```python
from build123d import *

# Parameters (mm, degrees)
SKETCH1_W           = 50
SKETCH1_H           = 9
SKETCH1_W_2         = 9
SKETCH1_H_2         = 68
BOSS_EXTRUDE1_DEPTH = 28
SKETCH2_R           = 2.5
CUT_EXTRUDE2_DEPTH  = 100
SKETCH4_R           = 4.5
CUT_EXTRUDE3_DEPTH  = 10
SKETCH5_R           = 10
CUT_EXTRUDE4_DEPTH  = 6
SKETCH7_R           = 1.5
CUT_EXTRUDE5_DEPTH  = 10
CUT_EXTRUDE6_DEPTH  = 10


with BuildPart() as part:
    # Sketch1 → Boss-Extrude1 (new body)
    with BuildSketch(Plane.XY):
        with Locations((-32.879310345, 31.301724138)):
            Rectangle(SKETCH1_W, SKETCH1_H)
        with Locations((-3.379310345, 1.801724138)):
            Rectangle(SKETCH1_W_2, SKETCH1_H_2)
        with Locations((-32.879310345, -27.698275862)):
            Rectangle(SKETCH1_W, SKETCH1_H)
    extrude(amount=BOSS_EXTRUDE1_DEPTH)

    # Sketch2 → Cut-Extrude2 (cut)
    with BuildSketch(Plane(origin=(0, 35.801724138, 0), x_dir=(1, 0, 0), z_dir=(0, 1, 0))):
        with Locations(Location((-43.879310345, -14, 0), (0, 0, 180))):
            Circle(SKETCH2_R)
        with BuildLine():
            ThreePointArc((-43.879310345, -28), (-53.778805281, -23.899494937), (-57.879310345, -14))
            Line((-57.879310345, -14), (-57.879310345, -28))
            Line((-57.879310345, -28), (-43.879310345, -28))
        make_face()
        with BuildLine():
            Line((-57.879310345, 0), (-57.879310345, -14))
            ThreePointArc((-57.879310345, -14), (-53.778805281, -4.100505063), (-43.879310345, 0))
            Line((-43.879310345, 0), (-57.879310345, 0))
        make_face()
    extrude(amount=-CUT_EXTRUDE2_DEPTH, mode=Mode.SUBTRACT)

    # Sketch4 → Cut-Extrude3 (cut)
    with BuildSketch(Plane(origin=(0, 35.801724138, 0), x_dir=(1, 0, 0), z_dir=(0, 1, 0))):
        with Locations(Location((-43.879310345, -14, 0), (0, 0, 180))):
            Circle(SKETCH4_R)
    extrude(amount=-CUT_EXTRUDE3_DEPTH, mode=Mode.SUBTRACT)

    # Sketch5 → Cut-Extrude4 (cut)
    with BuildSketch(Plane(origin=(0, 35.801724138, 0), x_dir=(1, 0, 0), z_dir=(0, 1, 0))):
        with Locations(Location((-43.879310345, -14, 0), (0, 0, 180))):
            Circle(SKETCH5_R)
    extrude(amount=-CUT_EXTRUDE4_DEPTH, mode=Mode.SUBTRACT)

    # Sketch7 → Cut-Extrude5 (cut)
    with BuildSketch(Plane(origin=(1.120689655, 0, 0), x_dir=(0, 0, -1), z_dir=(1, 0, 0))):
        with Locations(Location((-14, 8.801724138, 0), (0, 0, 90))):
            Circle(SKETCH7_R)
        with Locations(Location((-14, -5.198275862, 0), (0, 0, 90))):
            Circle(SKETCH7_R)
        with Locations(Location((-7, 1.801724138, 0), (0, 0, 90))):
            Circle(SKETCH7_R)
        with Locations(Location((-21, 1.801724138, 0), (0, 0, 90))):
            Circle(SKETCH7_R)
    extrude(amount=-CUT_EXTRUDE5_DEPTH, mode=Mode.SUBTRACT)

    # Sketch8 → Cut-Extrude6 (cut)
    with BuildSketch(Plane(origin=(0, 29.801724138, 0), x_dir=(1, 0, 0), z_dir=(0, 1, 0))):
        with BuildLine():
            ThreePointArc((-42.979310345, -21.003011395), (-43.242914242, -20.366615292), (-43.879310345, -20.103011395))
            Line((-43.879310345, -20.103011395), (-43.879310345, -21.903011395))
            ThreePointArc((-43.879310345, -21.903011395), (-43.242914242, -21.639407498), (-42.979310345, -21.003011395))
        make_face()
        with BuildLine():
            Line((-43.879310345, -21.903011395), (-43.879310345, -20.103011395))
            ThreePointArc((-43.879310345, -20.103011395), (-44.779310345, -21.003011395), (-43.879310345, -21.903011395))
        make_face()
        with BuildLine():
            ThreePointArc((-35.979310345, -14), (-36.879310345, -13.1), (-37.779310345, -14))
            Line((-37.779310345, -14), (-35.979310345, -14))
        make_face()
        with BuildLine():
            Line((-35.979310345, -14), (-37.779310345, -14))
            ThreePointArc((-37.779310345, -14), (-36.879310345, -14.9), (-35.979310345, -14))
        make_face()
        with BuildLine():
            ThreePointArc((-43.879310345, -6.1), (-44.779310345, -7), (-43.879310345, -7.9))
            Line((-43.879310345, -7.9), (-43.879310345, -6.1))
        make_face()
        with BuildLine():
            Line((-43.879310345, -6.1), (-43.879310345, -7.9))
            ThreePointArc((-43.879310345, -7.9), (-43.242914242, -7.636396103), (-42.979310345, -7))
            ThreePointArc((-42.979310345, -7), (-43.242914242, -6.363603897), (-43.879310345, -6.1))
        make_face()
        with BuildLine():
            ThreePointArc((-51.779310345, -14), (-50.879310345, -14.9), (-49.979310345, -14))
            Line((-49.979310345, -14), (-51.779310345, -14))
        make_face()
        with BuildLine():
            Line((-51.779310345, -14), (-49.979310345, -14))
            ThreePointArc((-49.979310345, -14), (-50.879310345, -13.1), (-51.779310345, -14))
        make_face()
    extrude(amount=-CUT_EXTRUDE6_DEPTH, mode=Mode.SUBTRACT)


solid = part.part
```
Part model, mm, in its own coordinate system. A direction names the side the tool comes from. Round coordinates to 2 decimals unless told otherwise and drop trailing zeros. Write each loop counter-clockwise with the first axis right and the second up, starting at its lowest first coordinate (ties: lowest second). Pieces come first, ordered by that corner, then holes. Notation, with made-up numbers: M -27.5,-31 L 25.5,-31 A17 ccw 25.5,-4 Z; hole C 4,89.25 d2. An arc over 180 degrees is marked long. One line per question, with ' | ' between items.
(1) Two-plate mould, pull along X, no slides. Class faces 1 (the face through (-3.316, -3.768, 14.451)), 2 (the face through (-7.879, 1, 14)), 3 (the face through (-41.895, -27.635, 12.479)): released by +X, released by -X, zero draft, split by the parting line, or undercut.
Answer key:
face 1: zero draft | face 2: released by -X | face 3: undercut
(2) Saw through at C-C on y = 5. Write the cut outline in (x, z), then the cut area to 3 significant figures.
Answer key:
outline: M -7.88,0 L 1.12,0 L 1.12,28 L -7.88,28 Z | area: 252 mm^2
(3) Pin check, flat tips, straight feed: pin 1 (1 mm diameter, centred on y = 5.5, z = 13, fed in from -X); pin 2 (3 mm diameter, centred on x = -36.88, z = 14, fed in from +Y). Stop position of each tip, or through.
Answer key:
pin 1: stops at x = -7.88 | pin 2: stops at y = 29.8
(4) Saw through at B-B on z = 25.75. Write the cut outline in (x, y), then the cut area to 3 significant figures.
Answer key:
outline: M -51.49,-32.2 L 1.12,-32.2 L 1.12,35.8 L -51.49,35.8 L -51.49,26.8 L -7.88,26.8 L -7.88,-23.2 L -51.49,-23.2 Z | area: 1,400 mm^2
(5) Saw through at A-A on x = -22.5. Write the cut outline in (y, z), then the cut area to 3 significant figures.
Answer key:
outline: M -32.2,0 L -23.2,0 L -23.2,28 L -32.2,28 Z; M 26.8,0 L 35.8,0 L 35.8,28 L 26.8,28 Z | area: 504 mm^2
(6) 3-axis set-ups, long thin cutter, end or side, ignore diameter. For faces 4 (the face through (-7, 2, 28)), 5 (the face through (-35.98, 28.32, 14.04)), 6 (the face through (-33, -23.198, 14)): which of +Z, -Z, +X, -X, +Y, -Y reach the whole face in a straight line?
Answer key:
face 4: +Z, +X, -X, +Y, -Y | face 5: +Y | face 6: +Z, -Z, -X
(7) Probe line 1 along Y through (x, z) = (-21, 9.5); line 2 along Y through (x, z) = (-51, 11.5); line 3 along X through (y, z) = (7, 24.75). List the from-to ranges inside material, lowest first.
Answer key:
line 1: y = -32.2 to -23.2, 26.8 to 35.8 | line 2: y = -32.2 to -23.2, 26.8 to 29.8 | line 3: x = -7.88 to 1.12
